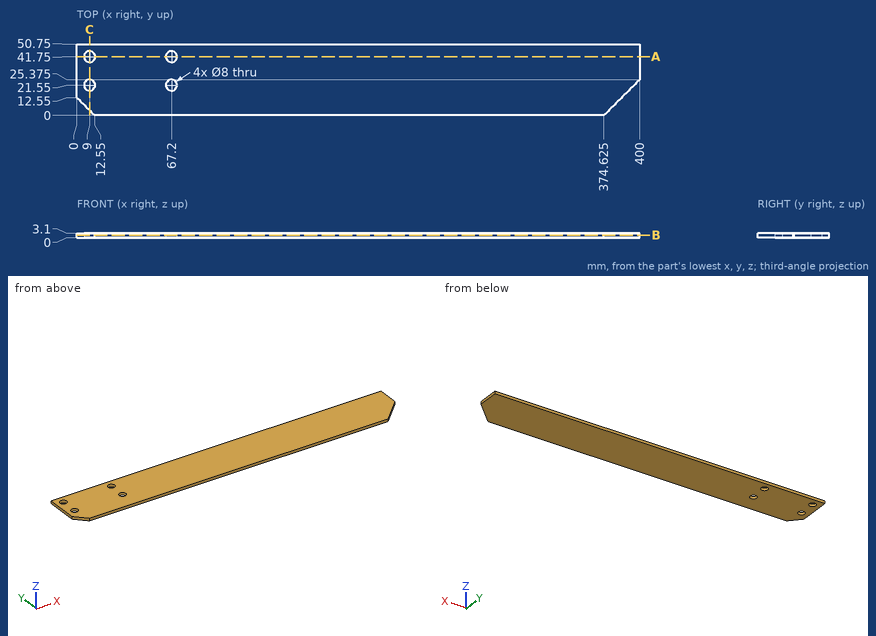
Can you work these out from the drawing? Everything is in mm from the part's minimum corner. Give positions to 0.01 mm unless a question says otherwise; leave off trailing zeros. Loops run counter-clockwise (first coordinate to the right, second up) from the corner with the lowest first, then second, coordinate; pieces in that order, holes last. Notation, with made-up numbers: M 36.25,27 L 62.25,27 A18 cw 62.25,36 Z; hole C 39.5,-35.75 d8. An arc over 180 degrees is marked long. Put each result on its own line as item: value. Start each with the question number.
(1) I want a section at B-B on z = 1.85. Please give me the cut outline in (x, y) (3 decimals).
(2) I want a section at C-C on x = 9. Please give me the cut outline in (y, z), then the cut area to 3 significant figures.
(3) I want a section at A-A on y = 41.75. Please give me the cut outline in (x, z), then the cut area to 3 significant figures.
(4) I need wall thicknesses on line 1 along Y through (x, z) = (67.2, 0.7); line 2 along X through (y, z) = (42, 0.4); line 3 along Y through (x, z) = (9, 2). Which ranges of each line are inside material? Lowest first, please. Write a range as [from, to].
Answer block:
1. outline: M 0,12.55 L 12.55,0 L 374.625,0 L 400,25.375 L 400,50.75 L 0,50.75 Z; hole C 9,21.55 d8; hole C 9,41.75 d8; hole C 67.2,21.55 d8; hole C 67.2,41.75 d8
2. outline: M 3.55,0 L 17.55,0 L 17.55,3.1 L 3.55,3.1 Z; M 25.55,0 L 37.75,0 L 37.75,3.1 L 25.55,3.1 Z; M 45.75,0 L 50.75,0 L 50.75,3.1 L 45.75,3.1 Z
2. area: 96.7 mm^2
3. outline: M 0,0 L 5,0 L 5,3.1 L 0,3.1 Z; M 13,0 L 63.2,0 L 63.2,3.1 L 13,3.1 Z; M 71.2,0 L 400,0 L 400,3.1 L 71.2,3.1 Z
3. area: 1,190 mm^2
4. line 1: [0, 17.55], [25.55, 37.75], [45.75, 50.75]
4. line 2: [0, 5.01], [12.99, 63.21], [71.19, 400]
4. line 3: [3.55, 17.55], [25.55, 37.75], [45.75, 50.75]
